Here's the drawing with two shaded views (mm, measured from the low corner). I have some questions. Round coordinates to 2 decimals unless told otherwise and drop trailing zeros. Order: outer loops, then holes, each group sorted by start corner. A loop starts at its lowest first (then second) coordinate and runs counter-clockwise, first axis right, second up.
Q1. We'd pull the mould along Y, two halves only. Please class the marked faces 1, 2 and 3: pulls with the +Y half, pulls with the -Y half, needs draft (parallel to the pull), parting line crosses it, or undercut.
Q2. Will these pins go through, and if not, where does the flat tip stop? P1, Ø3.5, axis at x = 34, z = 4.5, coming from the -Y side; P2, Ø6, axis at x = 17, y = 35.5, coming from the +Z side; P3, Ø2, axis at y = 50, z = 5, coming from the -X side; P4, Ø3, axis at y = 34.5, z = 7, coming from the -X side.
Q3. If we section it at C-C (y = 6): Please give me the cut outline in (x, z) (1 decimal).
Q4. If we section it at A-A (x = 80): Please give me the cut outline in (y, z).
Q5. If we section it at B-B (z = 2.75): Please give me the cut outline in (x, y) (1 decimal).
Q6. If I drill on line 1 (Y direction, x = 28, z = 2.5); line 2 (Z direction, x = 51, y = 47.5); line 3 (X direction, y = 3.5, z = 6.5) (1 decimal), over which ranges is the centre line in solid material (lowest first)?
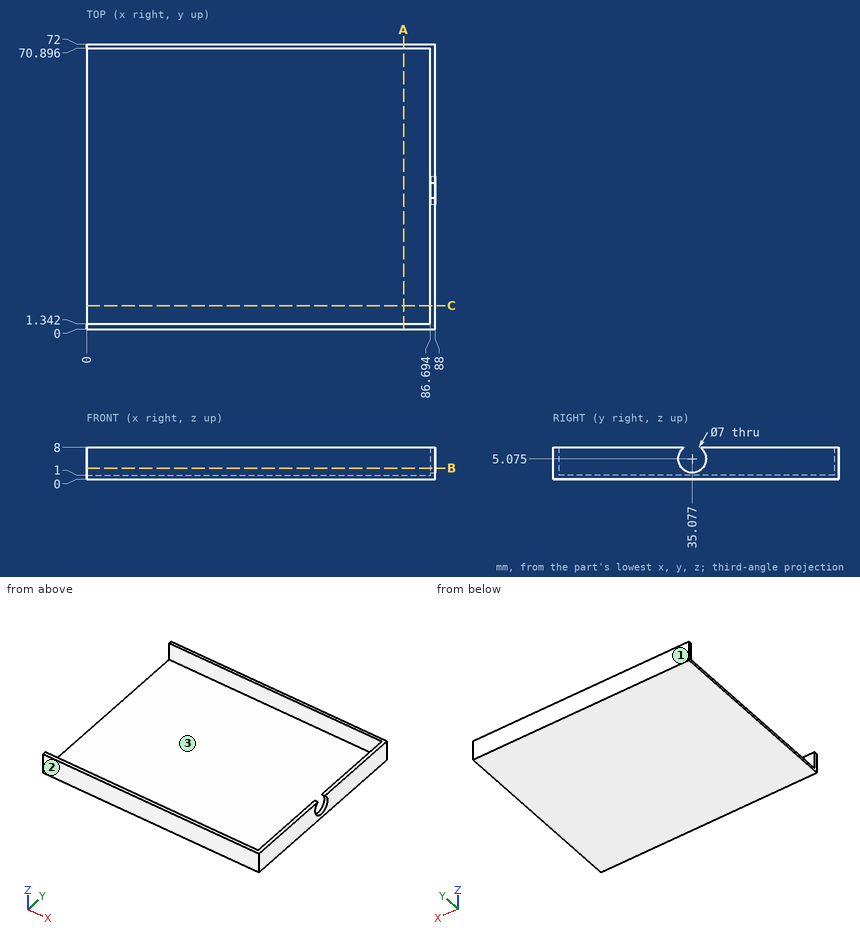
Solution:
1. face 1: pulls with the +Y half
1. face 2: pulls with the -Y half
1. face 3: undercut
2. P1: stops at y = 0
2. P2: stops at z = 1
2. P3: stops at x = 86.69
2. P4: passes through
3. outline: (0, 0) - (88, 0) - (88, 8) - (86.7, 8) - (86.7, 1) - (0, 1) - close
4. outline: (0, 0) - (72, 0) - (72, 8) - (70.9, 8) - (70.9, 1) - (1.34, 1) - (1.34, 8) - (0, 8) - close
5. outline: (0, 0) - (88, 0) - (88, 32.5) - (86.7, 32.5) - (86.7, 1.3) - (0, 1.3) - close; (0, 70.9) - (86.7, 70.9) - (86.7, 37.7) - (88, 37.7) - (88, 72) - (0, 72) - close
6. line 1: y = 0 to 1.34, 70.9 to 72
6. line 2: z = 0 to 1
6. line 3: x = 86.7 to 88
